Design review of the part built by this model. Coordinates are the model's own, in mm. A direction names the side the tool comes from. Round coordinates to 2 decimals unless told otherwise and drop trailing zeros. Order: outer loops, then holes, each group sorted by start corner. A loop starts at its lowest first (then second) coordinate and runs counter-clockwise, first axis right, second up. Notation, with made-up numbers: (81, 12.5) - (133, 12.5) arc R19 ccw to (133, 16.5) - close; hole circle Ø11 at (-10.75, 82.5). An arc over 180 degrees is marked (long way). Write item = value, one per line.
from build123d import *

# Parameters (mm, degrees)
SKETCH1_R           = 4.16
EXTRUDE1_DEPTH      = 11
SKETCH2_W           = 6.4
SKETCH2_H           = 6.357406019
EXTRUDE2_DEPTH      = 5.16
EXTRUDE2_DEPTH_BACK = 5.16
EXTRUDE3_DEPTH      = 5.16
EXTRUDE3_DEPTH_BACK = 5.16
SKETCH4_R           = 0.7
EXTRUDE4_DEPTH      = 5.1600001
EXTRUDE4_DEPTH_BACK = 5.1600001


with BuildPart() as part:
    # Sketch1 → Extrude1 (new body)
    with BuildSketch(Plane.XY):
        Circle(SKETCH1_R)
    extrude(amount=EXTRUDE1_DEPTH)

    # Sketch2 → Extrude2 (cut, two sides)
    with BuildSketch(Plane(origin=(0, 0, 0), x_dir=(1, 0, 0), z_dir=(0, 1, 0))) as extrude2_sk:
        with Locations((0, -8.67870301)):
            Rectangle(SKETCH2_W, SKETCH2_H)
    extrude(amount=EXTRUDE2_DEPTH, mode=Mode.SUBTRACT)
    extrude(extrude2_sk.sketch, amount=-EXTRUDE2_DEPTH_BACK, mode=Mode.SUBTRACT)

    # Sketch3 → Extrude3 (cut, two sides)
    with BuildSketch(Plane(origin=(0, 0, 0), x_dir=(0, 0, -1), z_dir=(1, 0, 0))) as extrude3_sk:
        with BuildLine():
            Line((-8.35, 2.65), (-8.35, 3.836721977))
            Line((-8.35, 3.836721977), (-12.822156105, 3.836721977))
            Line((-12.822156105, 3.836721977), (-12.822156105, -4.605164147))
            Line((-12.822156105, -4.605164147), (-8.35, -4.492230912))
            Line((-8.35, -4.492230912), (-8.35, -2.65))
            ThreePointArc((-8.35, -2.65), (-11, 0), (-8.35, 2.65))
        make_face()
    extrude(amount=EXTRUDE3_DEPTH, mode=Mode.SUBTRACT)
    extrude(extrude3_sk.sketch, amount=-EXTRUDE3_DEPTH_BACK, mode=Mode.SUBTRACT)

    # Sketch4 → Extrude4 (cut, two sides)
    with BuildSketch(Plane(origin=(0, 0, 0), x_dir=(0, 0, -1), z_dir=(1, 0, 0))) as extrude4_sk:
        with Locations((-9.1, 0)):
            Circle(SKETCH4_R)
    extrude(amount=EXTRUDE4_DEPTH, mode=Mode.SUBTRACT)
    extrude(extrude4_sk.sketch, amount=-EXTRUDE4_DEPTH_BACK, mode=Mode.SUBTRACT)


solid = part.part
1) Clearance check with flat-ended pins moving along their axes: pin 1 Ø4 at (x, z) = (-2, 6) entering from -Y; pin 2 Ø4 at (x, y) = (0.5, 1) entering from +Z; pin 3 Ø1 at (x, z) = (2, 2.5) entering from -Y. State where each tip first meets the part, or that it passes through.
Findings:
pin_1 = -4.16
pin_2 = 5.5
pin_3 = -3.88
2) To check wall thickness, follow L1, parallel to X at y = 0, z = 7.5; L2, parallel to Z at x = 3.7, y = 0; L3, parallel to Z at x = -1, y = -1.75. State the ranges of each line that lie inside material, in increasing order. Write a range as from..to.
Findings:
L1 = -4.16..-3.2, 3.2..4.16
L2 = 0..8.4, 9.8..11
L3 = 0..5.5
3) We need section A-A on y = 0. Write out the cut boundary in (x, z).
Findings:
outline = (-4.16, 0) - (4.16, 0) - (4.16, 8.4) - (3.2, 8.4) - (3.2, 5.5) - (-3.2, 5.5) - (-3.2, 8.4) - (-4.16, 8.4) - close; (-4.16, 9.8) - (-3.2, 9.8) - (-3.2, 11) - (-4.16, 11) - close; (3.2, 9.8) - (4.16, 9.8) - (4.16, 11) - (3.2, 11) - close
4) We need section B-B on z = 9.5. Write out the cut boundary in (x, y), and give its area (3 significant figures).
Findings:
outline = (-4.12, -0.57) arc R4.16 ccw to (-3.41, -2.39) - (-3.2, -2.39) - (-3.2, -0.57) - close; (-4.12, 0.57) - (-3.2, 0.57) - (-3.2, 2.39) - (-3.41, 2.39) arc R4.16 ccw to start; (3.2, -2.39) - (3.41, -2.39) arc R4.16 ccw to (4.12, -0.57) - (3.2, -0.57) - close; (3.2, 0.57) - (4.12, 0.57) arc R4.16 ccw to (3.41, 2.39) - (3.2, 2.39) - close
area = 4.69 mm^2
5) We need section D-D on x = 0. Write out the cut boundary in (y, z), and give its area (3 significant figures).
Findings:
outline = (-4.16, 0) - (4.16, 0) - (4.16, 5.5) - (-4.16, 5.5) - close
area = 45.8 mm^2
6) We need section C-C on z = 6. Write out the cut boundary in (x, y).
Findings:
outline = (-3.2, -2.66) - (-3.2, 2.66) arc R4.16 ccw to start; (3.2, -2.66) arc R4.16 ccw to (3.2, 2.66) - close
7) For faces 1 (the flat face through (-3.2, 0, 8)), 2 (the cylindrical face through (4, 0, 11)), list the 3-axis set-ups (+Z, -Z, +X, -X, +Y, -Y) from which the entire face can be reached by the end or side of a thin tool; tool diameter is ignored.
Findings:
face_1 = +Z, +Y, -Y
face_2 = +Z, +X, -X
8) The part is to be moulded in two halves that separate along Z. For faces 3 (the cylindrical face through (-3.7, 0, 9.8)), 4 (the cylindrical face through (-4, 0, 11)), 5 (the flat face through (3.2, 0, 8)), 6 (the cylindrical face through (3.7, 0, 9.8)), say which applies: released by +Z, released by -Z, zero draft, split by the parting line, or undercut.
Findings:
face_3 = undercut
face_4 = released by +Z
face_5 = zero draft
face_6 = undercut
